from build123d import *

# Parameters (mm, degrees)
SKETCH_1_R           = 4
EXTRUDE_1_DEPTH      = 17.8
SKETCH_2_R           = 1.9
EXTRUDE_2_DEPTH      = 1
SKETCH_3_R           = 1.9
EXTRUDE_3_DEPTH      = 1
SKETCH_4_R           = 4
EXTRUDE_4_DEPTH      = 6.45
EXTRUDE_4_DEPTH_BACK = 6.45
SKETCH_5_R           = 1.9
EXTRUDE_5_DEPTH      = 1
SKETCH_6_R           = 1.9
EXTRUDE_6_DEPTH      = 1


with BuildPart() as part:
    # Sketch 1 → Extrude 1 (new body)
    with BuildSketch(Plane.XY):
        Circle(SKETCH_1_R)
    extrude(amount=EXTRUDE_1_DEPTH)

    # Sketch 2 → Extrude 2 (add)
    with BuildSketch(Plane.XY.offset(17.8)):
        Circle(SKETCH_2_R)
    extrude(amount=EXTRUDE_2_DEPTH)

    # Sketch 3 → Extrude 3 (add)
    with BuildSketch(Plane(origin=(0, 0, 0), x_dir=(-1, 0, 0), z_dir=(0, 0, -1))):
        Circle(SKETCH_3_R)
    extrude(amount=EXTRUDE_3_DEPTH)

    # Sketch 4 → Extrude 4 (add, two sides)
    with BuildSketch(Plane(origin=(0, 0, 0), x_dir=(1, 0, 0), z_dir=(0, 1, 0))) as extrude_4_sk:
        with Locations((0, -8.9)):
            Circle(SKETCH_4_R)
    extrude(amount=EXTRUDE_4_DEPTH)
    extrude(extrude_4_sk.sketch, amount=-EXTRUDE_4_DEPTH_BACK)

    # Sketch 5 → Extrude 5 (add)
    with BuildSketch(Plane(origin=(0, -6.45, 0), x_dir=(-1, 0, 0), z_dir=(0, -1, 0))):
        with Locations((0, -8.9)):
            Circle(SKETCH_5_R)
    extrude(amount=EXTRUDE_5_DEPTH)

    # Sketch 6 → Extrude 6 (add)
    with BuildSketch(Plane(origin=(0, 6.45, 0), x_dir=(1, 0, 0), z_dir=(0, 1, 0))):
        with Locations((0, -8.9)):
            Circle(SKETCH_6_R)
    extrude(amount=EXTRUDE_6_DEPTH)


solid = part.part
Build history of the part. All positions in model axes, mm. A direction names the side the tool comes from. Give positions to 0.01 mm unless a question says otherwise; leave off trailing zeros. Loops run counter-clockwise (first coordinate to the right, second up) from the corner with the lowest first, then second, coordinate; pieces in that order, holes last. Notation, with made-up numbers: (6.5, -16.5) - (61.5, -16.5) arc R18 ccw to (61.5, -3.5) - close; hole circle Ø10 at (88, 35.5). An arc over 180 degrees is marked (long way). Write item = value, one per line. Start each with the question number.
1) Band-saw the part on B-B on y = 1. Give the cut face in (x, z).
2) Drop flat-ended pins along their axis: pin 1 Ø1 at (x, y) = (-2, -1) entering from -Z; pin 2 Ø4 at (y, z) = (5, 1.5) entering from +X; pin 3 Ø3 at (x, z) = (-1, 2.5) entering from -Y. Give the stop position or say it passes through.
3) Band-saw the part on D-D on y = -2.5. Give the cut face in (x, z).
4) Band-saw the part on C-C on z = 6.25. Give the cut face in (x, y).
5) Probe probe 1 along Y at (x, z) = (-2.5, 11.5); probe 2 along Z at (x, y) = (1.75, 1.75); probe 3 along Z at (x, y) = (1, -5.25). List the from-to ranges inside material, lowest first. Write a range as from..to.
6) Band-saw the part on A-A on x = 0. Give the cut face in (y, z).
7) Tool access for faces 1 (the cylindrical face through (-0.877, -6.943, 10.586)), 2 (the flat face through (0, 0, -1)), 3 (the flat face through (2, 6.45, 10)), 4 (the cylindrical face through (-1.9, 0.08, 18.29)), 5 (the cylindrical face through (1.9, 0.08, -0.49)): list every direction of +Z, -Z, +X, -X, +Y, -Y with a clear straight run to the whole face (end or side of a thin tool).
Final values:
q1.outline = (-3.87, 0) - (-1.62, 0) - (-1.62, -1) - (1.62, -1) - (1.62, 0) - (3.87, 0) - (3.87, 7.9) arc R4 ccw to (3.87, 9.9) - (3.87, 17.8) - (1.62, 17.8) - (1.62, 18.8) - (-1.62, 18.8) - (-1.62, 17.8) - (-3.87, 17.8) - (-3.87, 9.9) arc R4 ccw to (-3.87, 7.9) - close
q2.pin_1 = -1
q2.pin_2 = 2.65
q2.pin_3 = -4
q3.outline = (-3.12, 0) - (3.12, 0) - (3.12, 6.4) arc R4 ccw to (3.12, 11.4) - (3.12, 17.8) - (-3.12, 17.8) - (-3.12, 11.4) arc R4 ccw to (-3.12, 6.4) - close
q4.outline = (-3, -6.45) - (3, -6.45) - (3, -2.65) arc R4 ccw to (3, 2.65) - (3, 6.45) - (-3, 6.45) - (-3, 2.65) arc R4 ccw to (-3, -2.65) - close
q5.probe_1 = -6.45..6.45
q5.probe_2 = 0..17.8
q5.probe_3 = 5.03..12.77
q6.outline = (-7.45, 7) - (-6.45, 7) - (-6.45, 4.9) - (-4, 4.9) - (-4, 0) - (-1.9, 0) - (-1.9, -1) - (1.9, -1) - (1.9, 0) - (4, 0) - (4, 4.9) - (6.45, 4.9) - (6.45, 7) - (7.45, 7) - (7.45, 10.8) - (6.45, 10.8) - (6.45, 12.9) - (4, 12.9) - (4, 17.8) - (1.9, 17.8) - (1.9, 18.8) - (-1.9, 18.8) - (-1.9, 17.8) - (-4, 17.8) - (-4, 12.9) - (-6.45, 12.9) - (-6.45, 10.8) - (-7.45, 10.8) - close
q7.face_1 = -Y
q7.face_2 = -Z, +X, -X, +Y, -Y
q7.face_3 = +Y
q7.face_4 = +Z
q7.face_5 = -Z
